from build123d import *

# Parameters (mm, degrees)
SKETCH1_R                                      = 88.9
BOSS_EXTRUDE1_DEPTH                            = 6.35
CSK_FOR_8_FLAT_HEAD_MACHINE_SCREW1_D           = 4.4958
CSK_FOR_8_FLAT_HEAD_MACHINE_SCREW1_CSINK_D     = 9.7576132
CSK_FOR_8_FLAT_HEAD_MACHINE_SCREW1_CSINK_ANGLE = 82
CIRPATTERN1_COUNT                              = 2
SKETCH4_R                                      = 45.085
CUT_EXTRUDE1_DEPTH                             = 126.88384527
CUT_EXTRUDE2_DEPTH                             = 126.88384527
FILLET1_R                                      = 3.175
CIRPATTERN2_COUNT                              = 4
FILLET1_OF_CIRPATTERN2_R                       = 3.175


with BuildPart() as part:
    # Sketch1 → Boss-Extrude1 (new body)
    with BuildSketch(Plane(origin=(0, 0, 0), x_dir=(1, 0, 0), z_dir=(0, 1, 0))):
        with Locations(Location((0, 0, 0), (0, 0, 270))):
            Circle(SKETCH1_R)
    extrude(amount=BOSS_EXTRUDE1_DEPTH)

    # CSK for #8 Flat Head Machine Screw1 (through all)
    with Locations(Plane(origin=(0, 6.35, 0), x_dir=(-1, 0, 0), z_dir=(0, 1, 0))):
        with Locations((36.5125, -54.61), (-36.5125, -54.61), (36.5125, 54.61), (-36.5125, 54.61), (-54.61, -36.5125), (-54.61, 36.5125), (54.61, 36.5125), (54.61, -36.5125)):
            csk_for_8_flat_head_machine_screw1 = CounterSinkHole(CSK_FOR_8_FLAT_HEAD_MACHINE_SCREW1_D / 2, CSK_FOR_8_FLAT_HEAD_MACHINE_SCREW1_CSINK_D / 2, counter_sink_angle=CSK_FOR_8_FLAT_HEAD_MACHINE_SCREW1_CSINK_ANGLE)

    # CirPattern1: CSK for #8 Flat Head Machine Screw1 ×2 about axis
    cirpattern1_axis = Axis((0, 0, 0), (0, 1, 0))
    for i in range(1, CIRPATTERN1_COUNT):
        add(csk_for_8_flat_head_machine_screw1.rotate(cirpattern1_axis, i * 360 / CIRPATTERN1_COUNT), mode=Mode.SUBTRACT)

    # Sketch4 → Cut-Extrude1 (cut, through all)
    with BuildSketch(Plane(origin=(0, 6.35, 0), x_dir=(1, 0, 0), z_dir=(0, 1, 0))):
        with Locations(Location((0, 0, 0), (0, 0, 270))):
            Circle(SKETCH4_R)
    extrude(amount=-CUT_EXTRUDE1_DEPTH, mode=Mode.SUBTRACT)

    # Sketch5 → Cut-Extrude2 (cut, through all)
    with BuildSketch(Plane(origin=(0, 6.35, 0), x_dir=(1, 0, 0), z_dir=(0, 1, 0))):
        with BuildLine():
            Line((-68.817101203, -32.720736269), (-46.451543312, -22.086496982))
            ThreePointArc((-46.451543312, -22.086496982), (-51.435, 0), (-46.451543312, 22.086496982))
            Line((-46.451543312, 22.086496982), (-68.817101203, 32.720736269))
            ThreePointArc((-68.817101203, 32.720736269), (-76.2, 0), (-68.817101203, -32.720736269))
        make_face()
    cut_extrude2 = extrude(amount=-CUT_EXTRUDE2_DEPTH, mode=Mode.SUBTRACT)

    # Fillet1
    fillet1_edges = [part.edges().sort_by_distance(p)[0] for p in [
        (-68.817101203, 3.175, 32.720736269),
        (-68.817101203, 3.175, -32.720736269),
        (-46.451543312, 3.175, -22.086496982),
        (-46.451543312, 3.175, 22.086496982),
    ]]
    fillet(fillet1_edges, radius=FILLET1_R)

    # CirPattern2: Cut-Extrude2 ×4 about axis
    cirpattern2_axis = Axis((0, 0, 0), (0, 1, 0))
    for i in range(1, CIRPATTERN2_COUNT):
        add(cut_extrude2.rotate(cirpattern2_axis, i * 360 / CIRPATTERN2_COUNT), mode=Mode.SUBTRACT)

    # Fillet1 of CirPattern2
    fillet1_of_cirpattern2_edges = [part.edges().sort_by_distance(p)[0] for p in [
        (32.720736269, 3.175, 68.817101203),
        (-32.720736269, 3.175, 68.817101203),
        (-22.086496982, 3.175, 46.451543312),
        (22.086496982, 3.175, 46.451543312),
        (68.817101203, 3.175, -32.720736269),
        (68.817101203, 3.175, 32.720736269),
        (46.451543312, 3.175, 22.086496982),
        (46.451543312, 3.175, -22.086496982),
        (-32.720736269, 3.175, -68.817101203),
        (32.720736269, 3.175, -68.817101203),
        (22.086496982, 3.175, -46.451543312),
        (-22.086496982, 3.175, -46.451543312),
    ]]
    fillet(fillet1_of_cirpattern2_edges, radius=FILLET1_OF_CIRPATTERN2_R)


solid = part.part
Could you check a few things on this model? Use its own coordinates, in mm. A direction names the side the tool comes from. Give positions to 0.01 mm unless a question says otherwise; leave off trailing zeros. Order: outer loops, then holes, each group sorted by start corner. A loop starts at its lowest first (then second) coordinate and runs counter-clockwise, first axis right, second up.
1. Suppose I cut it at D-D (z = -54.61). List the corners of the cut face in (x, y) for me.
2. For faces 1 (the cylindrical face through (0.278, 3.219, 51.434)), 2 (the conical face through (54.3, 3.47, -34.16)), which set-ups out of +Z, -Z, +X, -X, +Y, -Y let a thin tool reach every point of the face, with its end or its side?
3. We'd pull the mould along Z, two halves only. Please class faces 3 (the cylindrical face through (34.267, 1.638, 54.709)), 4 (the flat face through (21, 0, -41)): pulls with the +Z half, pulls with the -Z half, needs draft (parallel to the pull), parting line crosses it, or undercut.
4. Will these pins go through, and if not, where does the flat tip stop? P1, Ø5, axis at x = -54.61, z = -36.51, coming from the +Y side; P2, Ø2, axis at x = 47.5, y = 2, coming from the -Z side; P3, Ø7, axis at x = -36.51, z = -54.61, coming from the +Y side.
5. Suppose I cut it at A-A (z = 0). List the corners of the cut face in (x, y) for me (3 decimals).
6. Suppose I cut it at B-B (x = -14.5). List the corners of the cut face in (y, z) for me, plus the area to 3 significant figures.
7. Suppose I cut it at C-C (y = 2.25). Give the number of separate pieces and of enclosed holes in the cut face, plus the area to 3 significant figures.
8. I need wall thicknesses on L1, parallel to Z at x = -54.61, y = 0.75; L2, parallel to Z at x = -17.5, y = 4.5; L3, parallel to X at y = 2, z = -27.5. Which ranges of each line are inside material? Lowest first, please.
Solved:
1. outline: (-70.15, 0) - (-38.76, 0) - (-38.76, 3.32) - (-41.39, 6.35) - (-70.15, 6.35) - close; (-34.26, 0) - (-25.97, 0) - (-25.97, 6.35) - (-31.63, 6.35) - (-34.26, 3.32) - close; (25.97, 0) - (34.26, 0) - (34.26, 3.32) - (31.63, 6.35) - (25.97, 6.35) - close; (38.76, 0) - (70.15, 0) - (70.15, 6.35) - (41.39, 6.35) - (38.76, 3.32) - close
2. face 1: +Y, -Y
2. face 2: +Y
3. face 3: undercut
3. face 4: needs draft
4. P1: stops at y = 3.62
4. P2: stops at z = -75.77
4. P3: stops at y = 4.77
5. outline: (-88.9, 0) - (-76.2, 0) - (-76.2, 6.35) - (-88.9, 6.35) - close; (-51.435, 0) - (-45.085, 0) - (-45.085, 6.35) - (-51.435, 6.35) - close; (45.085, 0) - (51.435, 0) - (51.435, 6.35) - (45.085, 6.35) - close; (76.2, 0) - (88.9, 0) - (88.9, 6.35) - (76.2, 6.35) - close
6. outline: (0, -87.71) - (6.35, -87.71) - (6.35, -74.81) - (0, -74.81) - close; (0, -49.35) - (6.35, -49.35) - (6.35, -42.69) - (0, -42.69) - close; (0, 42.69) - (6.35, 42.69) - (6.35, 49.35) - (0, 49.35) - close; (0, 74.81) - (6.35, 74.81) - (6.35, 87.71) - (0, 87.71) - close
6. area: 248 mm2
7. separate pieces: 1
7. enclosed holes: 13
7. area: 12,700 mm2
8. L1: z = -70.15 to -38.76, -34.26 to -25.97, 25.97 to 34.26, 38.76 to 70.15
8. L2: z = -87.16 to -74.16, -48.37 to -41.55, 41.55 to 48.37, 74.16 to 87.16
8. L3: x = -84.54 to -71.06, -57.84 to -35.73, 35.73 to 57.84, 71.06 to 84.54
